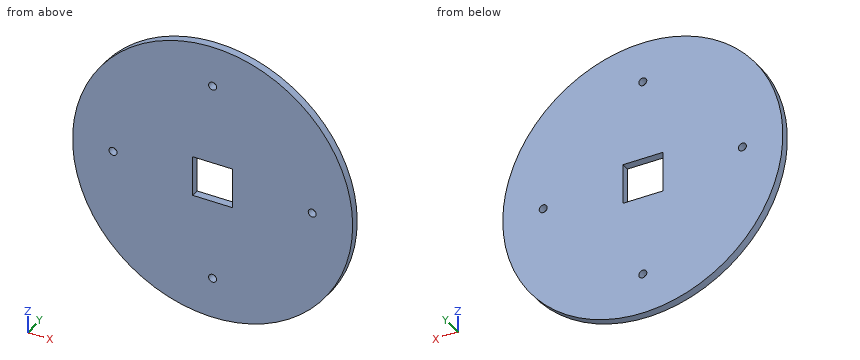
from build123d import *

# Parameters (mm, degrees)
SKETCH1_R           = 35
SKETCH1_R_2         = 1
SKETCH1_W           = 10
SKETCH1_H           = 10
BOSS_EXTRUDE1_DEPTH = 2


with BuildPart() as part:
    # Sketch1 → Boss-Extrude1 (new body)
    with BuildSketch(Plane(origin=(0, 0, 0), x_dir=(1, 0, 0), z_dir=(0, 1, 0))):
        Circle(SKETCH1_R)
        with Locations((0, 24.89)):
            Circle(SKETCH1_R_2, mode=Mode.SUBTRACT)
        with Locations((24.89, 0)):
            Circle(SKETCH1_R_2, mode=Mode.SUBTRACT)
        with Locations((0, -24.89)):
            Circle(SKETCH1_R_2, mode=Mode.SUBTRACT)
        with Locations((-24.89, 0)):
            Circle(SKETCH1_R_2, mode=Mode.SUBTRACT)
        Rectangle(SKETCH1_W, SKETCH1_H, mode=Mode.SUBTRACT)
    extrude(amount=BOSS_EXTRUDE1_DEPTH)


solid = part.part
Geometry check sheet. Reference: the model listing, model coordinates, mm. Round coordinates to 2 decimals unless told otherwise and drop trailing zeros. Write each loop counter-clockwise with the first axis right and the second up, starting at its lowest first coordinate (ties: lowest second). Pieces come first, ordered by that corner, then holes. Notation, with made-up numbers: (55, 10) -> (77, 10) arc R19 ccw to (77, 34) -> close; hole circle Ø6 at (66.5, -28). An arc over 180 degrees is marked (long way). One line per item, written item: value. Start each with the question number.
(1) Go/stop test with flat-tipped pins: pin 1 Ø0.6 at (y, z) = (1, 2.5) entering from +X; pin 2 Ø1.2 at (x, z) = (0, 24.89) entering from -Y; pin 3 Ø1 at (x, y) = (7, 0.5) entering from +Z; pin 4 Ø0.6 at (x, y) = (2, 0.5) entering from +Z. Record where each tip stops, or that it passes through.
(2) Cross-section at C-C, the plane y = 1.7. Record the cut outline in (x, z).
(3) Cross-section at D-D, the plane z = -24.89. Record the cut outline in (x, y), and give its area (3 significant figures).
(4) Cross-section at B-B, the plane x = -24.89. Record the cut outline in (y, z), and give its area (3 significant figures).
(5) Scan lines: line 1 (X direction, y = 1.1, z = 0); line 2 (Z direction, x = -24.89, y = 0.65). Record each from-to range of solid material in increasing order. Write a range as [from, to].
(6) Cross-section at A-A, the plane z = 0. Record the cut outline in (x, y), and give its area (3 significant figures).
Answer:
1. pin 1: x = 34.93
1. pin 2: through
1. pin 3: z = 34.39
1. pin 4: z = 34.96
2. outline: circle Ø70 at (0, 0); hole circle Ø2 at (-24.89, 0); hole (-5, -5) -> (5, -5) -> (5, 5) -> (-5, 5) -> close; hole circle Ø2 at (0, -24.89); hole circle Ø2 at (0, 24.89); hole circle Ø2 at (24.89, 0)
3. outline: (-24.61, 0) -> (-1, 0) -> (-1, 2) -> (-24.61, 2) -> close; (1, 0) -> (24.61, 0) -> (24.61, 2) -> (1, 2) -> close
3. area: 94.4 mm²
4. outline: (0, -24.61) -> (2, -24.61) -> (2, -1) -> (0, -1) -> close; (0, 1) -> (2, 1) -> (2, 24.61) -> (0, 24.61) -> close
4. area: 94.4 mm²
5. line 1: [-35, -25.89], [-23.89, -5], [5, 23.89], [25.89, 35]
5. line 2: [-24.61, -1], [1, 24.61]
6. outline: (-35, 0) -> (-25.89, 0) -> (-25.89, 2) -> (-35, 2) -> close; (-23.89, 0) -> (-5, 0) -> (-5, 2) -> (-23.89, 2) -> close; (5, 0) -> (23.89, 0) -> (23.89, 2) -> (5, 2) -> close; (25.89, 0) -> (35, 0) -> (35, 2) -> (25.89, 2) -> close
6. area: 112 mm²
